CAD build for the part. Positions are in the model's coordinates, mm. Face numbers are marked on the shaded views. Coordinates: 2 decimals unless noted, no trailing zeros. Loops run counter-clockwise (first coordinate to the right, second up) from the corner with the lowest first, then second, coordinate; pieces in that order, holes last. Notation, with made-up numbers: (44.25, 58.5) -> (58.25, 58.5) arc R11 cw to (58.25, 75.5) -> close; hole circle Ø11 at (26.5, 1). An arc over 180 degrees is marked (long way). Return JSON: item names as keys, results as strings. Group by question number.
(1) Saw through at C-C on x = 1.25. Write the cut outline in (y, z).
(2) Saw through at A-A on y = -1. Write the cut outline in (x, z).
(3) Saw through at B-B on z = -16. Write the cut outline in (x, y).
(4) Probe L1, parallel to X at y = -2.5, z = -8.5; L2, parallel to X at y = -0.5, z = -2; L3, parallel to Y at x = -0.25, z = 15.5. List the from-to ranges inside material, lowest first.
(5) Mould opens along X. For the marked faces 1, 2, 3 and 4 say: pulls with the +X half, pulls with the -X half, needs draft (parallel to the pull), parting line crosses it, or undercut.
(6) Saw through at D-D on x = -0.75. Write the cut outline in (y, z), then the cut area to 3 significant figures.
```python
from build123d import *

# Parameters (mm, degrees)
F0_W     = 12
F0_H     = 45
F1_DEPTH = 7
F2_R     = 3.25
F3_DEPTH = 45.001


with BuildPart() as f1:
    # F0 (on Front) → F1 (new body)
    with BuildSketch(Plane.XZ):
        Rectangle(F0_W, F0_H)
    extrude(amount=F1_DEPTH)

    # F2 (on face) → F3 (cut, through all)
    with BuildSketch(Plane.XY.offset(22.5)):
        Circle(F2_R)
    extrude(amount=-F3_DEPTH, mode=Mode.SUBTRACT)


solid = f1.part
```
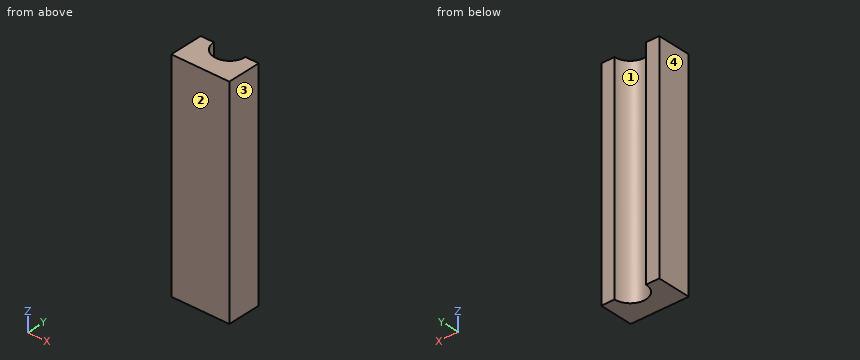
Geometry results:
{
 "1": {"outline": "(-7, -22.5) -> (-3, -22.5) -> (-3, 22.5) -> (-7, 22.5) -> close"},
 "2": {"outline": "(-6, -22.5) -> (-3.09, -22.5) -> (-3.09, 22.5) -> (-6, 22.5) -> close; (3.09, -22.5) -> (6, -22.5) -> (6, 22.5) -> (3.09, 22.5) -> close"},
 "3": {"outline": "(-6, -7) -> (6, -7) -> (6, 0) -> (3.25, 0) arc R3.25 cw to (-3.25, 0) -> (-6, 0) -> close"},
 "4": {"L1": "-6 to -2.08, 2.08 to 6", "L2": "-6 to -3.21, 3.21 to 6", "L3": "-7 to -3.24"},
 "5": {"face 1": "undercut", "face 2": "needs draft", "face 3": "pulls with the +X half", "face 4": "pulls with the -X half"},
 "6": {"outline": "(-7, -22.5) -> (-3.16, -22.5) -> (-3.16, 22.5) -> (-7, 22.5) -> close", "area": "173 mm²"}
}
